Build history of the part. All positions in model axes, mm. A direction names the side the tool comes from. Round coordinates to 2 decimals unless told otherwise and drop trailing zeros. Write each loop counter-clockwise with the first axis right and the second up, starting at its lowest first coordinate (ties: lowest second). Pieces come first, ordered by that corner, then holes. Notation, with made-up numbers: (-33.5, -7.75) - (-2.5, -7.75) arc R31 ccw to (-2.5, 21.25) - close; hole circle Ø11 at (56, -6). An arc over 180 degrees is marked (long way). One line per question, with ' | ' between items.
Autodesk Inventor part; units mm, degrees
ref_plane "YZ Plane" through (0, 0, 0) normal (1, 0, 0) x (0, 1, 0)
ref_plane "XZ Plane" through (0, 0, 0) normal (0, 1, 0) x (-1, 0, 0)
ref_plane "XY Plane" through (0, 0, 0) normal (0, 0, 1) x (1, 0, 0)
sketch "Sketch1" plane through (0, 0, 0) normal (0, 1, 0) x (-1, 0, 0)
  line L0 (0, 0) -> (9.8, 0)
  line L1 (9.8, 0) -> (9.8, -11.8)
  line L2 (9.8, -11.8) -> (0, -11.8)
  line L3 (0, -11.8) -> (0, 0)
  dimension "d0" = 11.8
  dimension "d1" = 9.8
extrude "Extrusion1" add sketch "Sketch1" along normal blind 8.8
sketch "Sketch2" plane through (0, 8.8, 0) normal (0, 1, 0) x (1, 0, 0)
  circle A0 centre (-4.9, 5.9) radius 1.4
  line L0 (-9.8, 0) -> (0, 0) construction
  line L1 (0, 0) -> (0, 11.8) construction
  line L2 (0, 11.8) -> (-9.8, 11.8) construction
  line L3 (-9.8, 11.8) -> (-9.8, 0) construction
  line L4 (0, 11.8) -> (-9.8, 11.8) construction
  line L5 (-4.9, 11.8) -> (-4.9, 0) construction
  line L6 (-9.8, 0) -> (0, 0) construction
  line L7 (-9.8, 11.8) -> (-9.8, 0) construction
  line L8 (-9.8, 5.9) -> (0, 5.9) construction
  line L9 (0, 0) -> (0, 11.8) construction
  line L10 (-5.9724, 6.8) -> (-3.8276, 6.8)
  point P0 (-4.9, 5.9)
  dimension "d4" = 2.8
  dimension "d5" = 0.9
extrude "Extrusion2" add sketch "Sketch2" along normal blind 10 contours A0 L10 picked at (-5.0611, 5.8774)
sketch "Sketch3" plane through (0, 0, 0) normal (0, -1, 0) x (1, 0, 0)
  line L0 (0, 0) -> (0, -11.8)
  line L1 (0, -2.4) -> (0, -9.4)
  line L2 (-9.8, -11.8) -> (-9.8, 0)
  line L3 (-9.8, -2.4) -> (-9.8, -9.4)
  arc A0 (0, -2.4) -> (-9.8, -2.4) centre (-4.9, -6.2021) ccw
  arc A1 (-9.8, -9.4) -> (0, -9.4) centre (-4.9, -5.5979) ccw
  line L4 (-9.8, 0) -> (0, 0)
  line L5 (0, -11.8) -> (-9.8, -11.8)
  point P0 (0, -5.9)
  point P1 (-9.8, -5.9)
  point P2 (-4.9, 0)
  point P3 (-4.9, -11.8)
  dimension "d8" = 7
  dimension "d9" = 7
extrude "Extrusion3" add sketch "Sketch3" along normal blind 14.5 contours L0 A1 L2 A0
sketch "Sketch4" plane through (0, -14.5, 0) normal (0, -1, 0) x (1, 0, 0)
  arc A0 (0, -2.4) -> (-9.8, -2.4) centre (-4.9, -6.2021) ccw
  line L0 (-9.8, -2.4) -> (-9.8, -9.4)
  arc A1 (-9.8, -9.4) -> (0, -9.4) centre (-4.9, -5.5979) ccw
  line L1 (0, -9.4) -> (0, -2.4)
  line L2 (-9.8, 0) -> (0, 0)
  line L3 (-4.9, 0) -> (7.2, 0)
  line L4 (7.2, 0) -> (7.2, -11.8)
  line L5 (7.2, -11.8) -> (-4.9, -11.8)
  line L6 (-4.9, -11.8) -> (-4.9, 0)
  dimension "d12" = 17
extrude "Extrusion4" add sketch "Sketch4" along normal blind 5
properties part number "moteur"
Q1. Drop flat-ended pins along their axis: pin 1 (1 mm diameter, centred on y = -2.5, z = -1.5, fed in from +X); pin 2 (2.5 mm diameter, centred on x = -5.5, y = 13, fed in from -Z); pin 3 (3 mm diameter, centred on x = 5, z = -7, fed in from +Y). Give the stop position or say it passes through.
Found:
pin 1: x = -0.34 | pin 2: z = -6.8 | pin 3: y = -14.5
Q2. Saw through at A-A, the plane z = -5.9. List the corners of the cut face in (x, y).
Found:
outline: (-9.8, -19.5) - (7.2, -19.5) - (7.2, -14.5) - (0, -14.5) - (0, 8.8) - (-3.5, 8.8) - (-3.5, 18.8) - (-6.3, 18.8) - (-6.3, 8.8) - (-9.8, 8.8) - close
Q3. Which spindle directions (+Z, -Z, +X, -X, +Y, -Y) get a long thin tool onto all of the face, cutting with end or side? Do faces 1 (the flat face through (-5, 14, -6.8)), 2 (the flat face through (-1, 0, -11)), 3 (the flat face through (-9, 0, -1)). Say none if no direction does.
Found:
face 1: -Z, +X, -X, +Y | face 2: -Z, +X | face 3: +Z, -X, -Y
Q4. Saw through at D-D, the plane z = -8.75. List the corners of the cut face in (x, y), then the cut area to 3 significant figures.
Found:
outline: (-9.8, -19.5) - (7.2, -19.5) - (7.2, -14.5) - (0, -14.5) - (0, 8.8) - (-9.8, 8.8) - close | area: 313 mm^2
Q5. Saw through at B-B, the plane y = -3.5. List the corners of the cut face in (x, z).
Found:
outline: (-9.8, -9.4) arc R6.2 ccw to (0, -9.4) - (0, -2.4) arc R6.2 ccw to (-9.8, -2.4) - close
Q6. Pull direction X, two halves, no side cores. Call faces 4 (the flat face through (-9.8, -2, -6)), 5 (the flat face through (0, 0, -6)), 6 (the flat face through (1, -17, -11.8)), 7 (the cylindrical face through (-5, -10, 0)): +X half, -X half, draft (parallel to the pull), parting line (faces both ways), or undercut.
Found:
face 4: -X half | face 5: +X half | face 6: draft | face 7: parting line
Q7. Drill centre lines: L1, parallel to Y at x = -1.25, z = -0.75; L2, parallel to Y at x = -4.5, z = -10; L3, parallel to Y at x = 3.75, z = -10. Where is each one in solid material? Low to high. Write a range as from..to.
Found:
L1: -19.5..-14.5, 0..8.8 | L2: -19.5..8.8 | L3: -19.5..-14.5
